Autodesk Inventor part; units mm, degrees
ref_plane "YZ Plane" through (0, 0, 0) normal (1, 0, 0) x (0, 1, 0)
ref_plane "XZ Plane" through (0, 0, 0) normal (0, 1, 0) x (-1, 0, 0)
ref_plane "XY Plane" through (0, 0, 0) normal (0, 0, 1) x (1, 0, 0)
sketch "Sketch1" plane through (0, 0, 0) normal (0, 0, 1) x (1, 0, 0)
  line L0 (-10, -10) -> (-5.6, -10)
  line L1 (-10, -5.6) -> (-10, -10)
  line L2 (-5.6, -10) -> (-5, -10)
  line L3 (-3.2, -8.2) -> (-5.6, -8.2)
  line L4 (-2.8351, -3.825) -> (-5.6, -6.5899)
  line L5 (-3.825, -2.8351) -> (-6.5899, -5.6)
  line L6 (0, 0) -> (0, -11) construction
  line L7 (0, 0) -> (-12, 0) construction
  line L8 (-3.2, -8.2) -> (-5, -10)
  line L9 (-6.5899, -5.6) -> (-8.2, -5.6)
  line L10 (-10, -5.6) -> (-10, -5)
  line L11 (-10, -5) -> (-8.2, -3.2)
  line L12 (-8.2, -3.2) -> (-8.2, -5.6)
  line L13 (-5.6, -8.2) -> (-5.6, -6.5899)
  arc A0 (-2.15, 0) -> (0, -2.15) centre (0, 0) ccw
  line L14 (0, 0) -> (-3.825, 0)
  line L15 (-3.825, 0) -> (-3.825, -2.8351)
  line L16 (-2.8351, -3.825) -> (0, -3.825)
  line L17 (0, -3.825) -> (0, 0)
  line L18 (-2.8351, -3.825) -> (-3.825, -3.825) construction
  line L19 (-3.825, -3.825) -> (-3.825, -2.8351) construction
  line L20 (3.825, -2.8351) -> (3.825, -3.825) construction
  line L21 (3.825, -2.8351) -> (3.825, 0)
  line L22 (3.825, -3.825) -> (2.8351, -3.825) construction
  line L23 (3.825, 0) -> (0, 0)
  line L24 (0, -3.825) -> (2.8351, -3.825)
  arc A1 (0, -2.15) -> (2.15, 0) centre (0, 0) ccw
  line L25 (0, 0) -> (0, -3.825)
  line L26 (2.8351, -3.825) -> (5.6, -6.5899)
  line L27 (0, 0) -> (0, -12) construction
  line L28 (0, 0) -> (11, 0) construction
  line L29 (3.825, -2.8351) -> (6.5899, -5.6)
  line L30 (8.2, -3.2) -> (8.2, -5.6)
  line L31 (10, -5.6) -> (10, -5)
  line L32 (8.2, -3.2) -> (10, -5)
  line L33 (8.2, -5.6) -> (6.5899, -5.6)
  line L34 (5.6, -6.5899) -> (5.6, -8.2)
  line L35 (10, -10) -> (10, -5.6)
  line L36 (5.6, -10) -> (10, -10)
  line L37 (3.2, -8.2) -> (5.6, -8.2)
  line L38 (5, -10) -> (3.2, -8.2)
  line L39 (5.6, -10) -> (5, -10)
  line L40 (2.8351, 3.825) -> (3.825, 3.825) construction
  line L41 (2.8351, 3.825) -> (0, 3.825)
  line L42 (3.825, 3.825) -> (3.825, 2.8351) construction
  line L43 (0, 3.825) -> (0, 0)
  line L44 (3.825, 0) -> (3.825, 2.8351)
  arc A2 (2.15, 0) -> (0, 2.15) centre (0, 0) ccw
  line L45 (0, 0) -> (3.825, 0)
  line L46 (3.825, 2.8351) -> (6.5899, 5.6)
  line L47 (0, 0) -> (12, 0) construction
  line L48 (0, 0) -> (0, 11) construction
  line L49 (2.8351, 3.825) -> (5.6, 6.5899)
  line L50 (3.2, 8.2) -> (5.6, 8.2)
  line L51 (5.6, 10) -> (5, 10)
  line L52 (3.2, 8.2) -> (5, 10)
  line L53 (5.6, 8.2) -> (5.6, 6.5899)
  line L54 (6.5899, 5.6) -> (8.2, 5.6)
  line L55 (10, 10) -> (5.6, 10)
  line L56 (10, 5.6) -> (10, 10)
  line L57 (8.2, 3.2) -> (8.2, 5.6)
  line L58 (10, 5) -> (8.2, 3.2)
  line L59 (10, 5.6) -> (10, 5)
  line L60 (-3.825, 2.8351) -> (-3.825, 3.825) construction
  line L61 (-3.825, 2.8351) -> (-3.825, 0)
  line L62 (-3.825, 3.825) -> (-2.8351, 3.825) construction
  line L63 (-3.825, 0) -> (0, 0)
  line L64 (0, 3.825) -> (-2.8351, 3.825)
  arc A3 (0, 2.15) -> (-2.15, 0) centre (0, 0) ccw
  line L65 (0, 0) -> (0, 3.825)
  line L66 (-2.8351, 3.825) -> (-5.6, 6.5899)
  line L67 (0, 0) -> (0, 12) construction
  line L68 (0, 0) -> (-11, 0) construction
  line L69 (-3.825, 2.8351) -> (-6.5899, 5.6)
  line L70 (-8.2, 3.2) -> (-8.2, 5.6)
  line L71 (-10, 5.6) -> (-10, 5)
  line L72 (-8.2, 3.2) -> (-10, 5)
  line L73 (-8.2, 5.6) -> (-6.5899, 5.6)
  line L74 (-5.6, 6.5899) -> (-5.6, 8.2)
  line L75 (-10, 10) -> (-10, 5.6)
  line L76 (-5.6, 10) -> (-10, 10)
  line L77 (-3.2, 8.2) -> (-5.6, 8.2)
  line L78 (-5, 10) -> (-3.2, 8.2)
  line L79 (-5.6, 10) -> (-5, 10)
  point P0 (0, 2.15)
  point P1 (2.15, 0)
  point P2 (0, -2.15)
  dimension "d16" = 10
  dimension "d19" = 3.2
  dimension "d21" = 4.4
  dimension "d22" = 4.4
  dimension "d24" = 45
  dimension "d25" = 1.8
  dimension "d27" = 1.8
  dimension "d28" = 45
  dimension "d29" = 3.2
  dimension "d31" = 1.4
  dimension "d33" = 2.15
  dimension "d34" = 3.825
  dimension "d35" = 3.825
  dimension "d36" = 135
  dimension "d39" = 360
extrude "ExtrusionModifier" add sketch "Sketch1" along normal blind 272.4 contours L1 L10 L11 L12 L9 L5 L15 L14 A0 L17 L16 L4 L13 L3 L8 L2 L0 | L17 A1 L23 L21 L29 L33 L30 L32 L31 L35 L36 L39 L38 L37 L34 L26 L24 | L61 L69 L73 L70 L72 L71 L75 L76 L79 L78 L77 L74 L66 L64 L43 A3 L14 | A2 L43 L41 L49 L53 L50 L52 L51 L55 L56 L59 L58 L57 L54 L46 L44 L23
pattern_linear "Rectangular Pattern1" count 2 spacing 20 along (0, -1, 0) of "ExtrusionModifier"
sketch "Sketch2" plane through (0, 0, 272.4) normal (0, 0, 1) x (1, 0, 0)
  line L0 (3.2, -8.2) -> (5, -10)
  line L1 (-3.2, -11.8) -> (-5, -10)
  line L2 (5, -10) -> (-5, -10) construction
  line L3 (-8.2, -12.25) -> (8.2, -12.25)
  line L4 (8.2, -12.25) -> (8.2, -7.75)
  line L5 (8.2, -7.75) -> (-8.2, -7.75)
  line L6 (-8.2, -7.75) -> (-8.2, -12.25)
  line L7 (-8.2, -12.25) -> (8.2, -7.75) construction
  line L8 (8.2, -12.25) -> (-8.2, -7.75) construction
  line L9 (10, -15) -> (10, -5)
  line L10 (5.6, -6.5899) -> (5.6, -8.2)
  line L11 (5.6, -6.5899) -> (6.7601, -7.75)
  line L12 (-5.6, -6.5899) -> (-2.8351, -3.825)
  line L13 (-5.6, -6.5899) -> (-6.7601, -7.75)
  line L14 (5.6, -13.4101) -> (6.7601, -12.25)
  line L15 (-5.6, -13.4101) -> (-6.7601, -12.25)
  line L16 (-5.6, -6.5899) -> (-5.6, -7.75)
  line L17 (-5.6, -8.2) -> (-5.6, -6.5899)
  line L18 (5.6, -6.5899) -> (5.6, -7.75)
  line L19 (-5.6, -11.8) -> (-5.6, -13.4101)
  line L20 (5.6, -13.4101) -> (5.6, -12.25)
  point P0 (0, 0)
  point P1 (0, -10)
  point P2 (-5.6, -12.25)
  dimension "d46" = 4.5
  dimension "d50" = 1.8
extrude "NoEdit" cut sketch "Sketch2" against normal through all
properties part number "AP20x20"
Geometry: final body of the model. Coordinates: model frame, mm. A direction names the side the tool comes from. Coordinates: 2 decimals unless noted, no trailing zeros. Use a Markdown table: item, result. Add a question column.
(1) Pin query (flat end, axial travel): pin 1 Ø4 at (x, z) = (4, 168.5) entering from +Y; pin 2 Ø1.2 at (y, z) = (-4, 109) entering from +X; pin 3 Ø4.5 at (x, z) = (1, 80.5) entering from +Y; pin 4 Ø1.5 at (x, z) = (-2, 46.5) entering from -Y (3 decimals). Return the tip coordinate at first contact, or that it passes through.
(2) Line query: line 1 along Y through (x, z) = (0, 55) (3 decimals); line 2 along Y through (x, z) = (-8.25, 106); line 3 along X through (y, z) = (0, 201) (3 decimals). Output: solid intervals per line, ascending.
(3) Access query for faces 1 (the flat face through (0, -23.825, 134)), 2 (the flat face through (0, -16.175, 134)), 3 (the flat face through (-3.825, 0, 134)), 4 (the flat face through (3.825, -20, 134)), 5 (the flat face through (10, 7, 134)). Directions: +Z, -Z, +X, -X, +Y, -Y. A direction counts if a zero-diameter tool reaches every point of the face in a straight line with its end or side. Return the directions, or none.
(4) Section query A-A, the plane z = 31.5. State how many separate pieces and enclosed holes the cut face has, plus the area to 3 significant figures.
(5) Mould query, pull axis X, two halves, no side actions, for faces 6 (the flat face through (-10, 8, 134)), 7 (the flat face through (-5, -5, 0)), 8 (the flat face through (10, -10, 134)), 9 (the flat face through (-8.2, -10, 138)). Classes: pulls with the +X half, pulls with the -X half, needs draft (parallel to the pull), parting line crosses it, or undercut.
Answer:
| question | item | result |
|---|---|---|
| 1 | pin 1 | stops at y = 10 |
| 1 | pin 2 | stops at x = 9.6 |
| 1 | pin 3 | stops at y = 8.25 |
| 1 | pin 4 | stops at y = -23.825 |
| 2 | line 1 | y = -23.825 to -22.15, -17.85 to -16.175, -3.825 to -2.15, 2.15 to 3.825 |
| 2 | line 2 | y = -30 to -23.25, -16.75 to -3.25, 3.25 to 10 |
| 2 | line 3 | x = -3.825 to -2.15, 2.15 to 3.825 |
| 3 | face 1 | +Z, -Z, -Y |
| 3 | face 2 | +Z, -Z |
| 3 | face 3 | +Z, -Z, -X |
| 3 | face 4 | +Z, -Z, +X |
| 3 | face 5 | +Z, -Z, +X, +Y, -Y |
| 4 | separate pieces | 1 |
| 4 | enclosed holes | 3 |
| 4 | area | 285 mm^2 |
| 5 | face 6 | pulls with the -X half |
| 5 | face 7 | needs draft |
| 5 | face 8 | pulls with the +X half |
| 5 | face 9 | undercut |
